Input: part model. Units: mm. Frame: model coordinates. Coordinates: 2 decimals unless noted, no trailing zeros. Loops run counter-clockwise (first coordinate to the right, second up) from the corner with the lowest first, then second, coordinate; pieces in that order, holes last. Notation, with made-up numbers: (17, 5) -> (62, 5) arc R21 ccw to (62, 43) -> close; hole circle Ø6 at (71.5, 75.25). An arc over 180 degrees is marked (long way). Answer as a JSON object with one key per item and string values.
Autodesk Inventor part; units mm, degrees
ref_plane "YZ Plane" through (0, 0, 0) normal (1, 0, 0) x (0, 1, 0)
ref_plane "XZ Plane" through (0, 0, 0) normal (0, 1, 0) x (-1, 0, 0)
ref_plane "XY Plane" through (0, 0, 0) normal (0, 0, 1) x (1, 0, 0)
sketch "Sketch1" plane through (0, 0, 0) normal (0, 0, 1) x (1, 0, 0)
  line L0 (-6.6675, 0) -> (6.6675, 0)
  line L1 (0, -6.35) -> (0, 4.7625)
  line L2 (-3.175, 3.175) -> (-3.175, -3.175)
  line L3 (-3.175, -3.175) -> (3.175, -3.175)
  line L4 (3.175, -3.175) -> (3.175, 3.175)
  line L5 (4.7625, 3.175) -> (4.7625, -4.7625)
  line L6 (4.7625, -4.7625) -> (-4.7625, -4.7625)
  line L7 (-4.7625, -4.7625) -> (-4.7625, 3.175)
  line L8 (-3.175, 3.175) -> (-4.7625, 3.175)
  line L9 (3.175, 3.175) -> (4.7625, 3.175)
  point P0 (0, 0)
  point P1 (0, -3.175)
  point P2 (-3.175, 0)
  dimension "d0" = 1.5875
  dimension "d1" = 6.35
  dimension "d2" = 6.35
extrude "Extrusion1" add sketch "Sketch1" along normal mid plane 600.075 contours L7 L8 L2 L0 | L0 L2 L3 L1 L6 L7 | L1 L3 L4 L0 L5 L6 | L4 L9 L5 L0
sketch "Sketch2" plane through (4.7625, -4.7625, 300.0375) normal (1, 0, 0) x (0, 0, -1)
  line L0 (0, 7.9375) -> (0, 0)
  line L1 (0, 0) -> (600.075, 0)
  line L2 (0, 7.9375) -> (600.075, 7.9375)
  line L3 (0, 0) -> (7.9375, 7.9375)
  line L4 (7.9375, 7.9375) -> (0, 7.9375)
  line L5 (0, 7.9375) -> (0, 0)
  line L6 (300.0375, 0) -> (300.0375, 7.9375) construction
  line L7 (600.075, 7.9375) -> (600.075, 0)
  line L8 (600.075, 0) -> (592.1375, 7.9375)
  line L9 (600.075, 7.9375) -> (592.1375, 7.9375)
  line L10 (7.9375, 7.9375) -> (0, 7.9375)
  point P0 (300.0375, 4.7625)
  dimension "d5" = 45
extrude "Extrusion2" cut sketch "Sketch2" against normal through all contours L2 L3 L0 | L8 L2 L7
properties part number "c-channel template" material "Aluminum-6061"
1. Section query B-B (z = 148.5). Return loops of the section in (x, y) (1 decimal), plus the area to 3 significant figures.
Reply:
{"outline": "(-4.8, -4.8) -> (4.8, -4.8) -> (4.8, 3.2) -> (3.2, 3.2) -> (3.2, -3.2) -> (-3.2, -3.2) -> (-3.2, 3.2) -> (-4.8, 3.2) -> close", "area": "35.3 mm2"}
2. Pin query (flat end, axial travel): P1, Ø1.5, axis at x = -3, y = -3.5, coming from the +Z side (3 decimals); P2, Ø1, axis at x = -1, z = 83.5, coming from the +Y side (3 decimals). Return the tip coordinate at first contact, or that it passes through.
Reply:
{"P1": "stops at z = 299.525", "P2": "stops at y = -3.175"}
3. Section query A-A (y = -1). Return loops of the section in (x, z) (1 decimal), plus the area to 3 significant figures.
Reply:
{"outline": "(-4.8, -296.3) -> (-3.2, -296.3) -> (-3.2, 296.3) -> (-4.8, 296.3) -> close; (3.2, -296.3) -> (4.8, -296.3) -> (4.8, 296.3) -> (3.2, 296.3) -> close", "area": "1,880 mm2"}
4. Line query: line 1 along X through (y, z) = (-2.5, -189) (1 decimal); line 2 along Y through (x, z) = (-1.75, 162.5) (1 decimal); line 3 along Z through (x, y) = (-0.5, -4.5) (3 decimals). Output: solid intervals per line, ascending.
Reply:
{"line 1": "x = -4.8 to -3.2, 3.2 to 4.8", "line 2": "y = -4.8 to -3.2", "line 3": "z = -299.775 to 299.775"}
